Can you work these out from the model? Positions are in its coordinate system, mm. A direction names the side the tool comes from. Coordinates: 2 decimals unless noted, no trailing zeros. Order: outer loops, then holes, each group sorted by start corner. A loop starts at its lowest first (then second) coordinate and runs counter-clockwise, first axis right, second up. Notation, with made-up numbers: (-15.75, -4.5) -> (-6.75, -4.5) arc R17 cw to (-6.75, 9.5) -> close; hole circle Ø6 at (-9, 17.5). An arc over 180 degrees is marked (long way). Answer in a Markdown table with one row per item.
```python
from build123d import *

# Parameters (mm, degrees)
BOSS_EXTRUDE1_DEPTH = 23.622
BOSS_EXTRUDE2_DEPTH = 10.668
SKETCH4_R           = 1.499997
BOSS_EXTRUDE3_DEPTH = 8


with BuildPart() as part:
    # Sketch1 → Boss-Extrude1 (new body)
    with BuildSketch(Plane(origin=(0, 0, 0), x_dir=(1, 0, 0), z_dir=(0, 1, 0))):
        with BuildLine():
            Line((11.557, 4.953), (-11.557, 4.953))
            ThreePointArc((-11.557, 4.953), (-11.916210245, 4.804210245), (-12.065, 4.445))
            Line((-12.065, 4.445), (-12.065, -4.445))
            ThreePointArc((-12.065, -4.445), (-11.916210245, -4.804210245), (-11.557, -4.953))
            Line((-11.557, -4.953), (11.557, -4.953))
            ThreePointArc((11.557, -4.953), (11.916210245, -4.804210245), (12.065, -4.445))
            Line((12.065, -4.445), (12.065, 4.445))
            ThreePointArc((12.065, 4.445), (11.916210245, 4.804210245), (11.557, 4.953))
        make_face()
    extrude(amount=BOSS_EXTRUDE1_DEPTH)

    # Sketch2 → Boss-Extrude2 (add)
    with BuildSketch(Plane(origin=(0, 23.622, 0), x_dir=(1, 0, 0), z_dir=(0, 1, 0))):
        with BuildLine():
            Line((11.557, 4.953), (-11.557, 4.953))
            ThreePointArc((-11.557, 4.953), (-11.916210245, 4.804210245), (-12.065, 4.445))
            Line((-12.065, 4.445), (-12.065, -4.445))
            ThreePointArc((-12.065, -4.445), (-11.916210245, -4.804210245), (-11.557, -4.953))
            Line((-11.557, -4.953), (11.557, -4.953))
            ThreePointArc((11.557, -4.953), (11.916210245, -4.804210245), (12.065, -4.445))
            Line((12.065, -4.445), (12.065, 4.445))
            ThreePointArc((12.065, 4.445), (11.916210245, 4.804210245), (11.557, 4.953))
        make_face()
        with BuildLine():
            Line((10.287, -3.683), (-10.287, -3.683))
            ThreePointArc((-10.287, -3.683), (-10.646210245, -3.534210245), (-10.795, -3.175))
            Line((-10.795, -3.175), (-10.795, 3.175))
            ThreePointArc((-10.795, 3.175), (-10.646210245, 3.534210245), (-10.287, 3.683))
            Line((-10.287, 3.683), (10.287, 3.683))
            ThreePointArc((10.287, 3.683), (10.646210245, 3.534210245), (10.795, 3.175))
            Line((10.795, 3.175), (10.795, -3.175))
            ThreePointArc((10.795, -3.175), (10.646210245, -3.534210245), (10.287, -3.683))
        make_face(mode=Mode.SUBTRACT)
    extrude(amount=BOSS_EXTRUDE2_DEPTH)

    # Sketch4 → Boss-Extrude3 (add)
    with BuildSketch(Plane(origin=(0, 0, 0), x_dir=(1, 0, 0), z_dir=(0, 1, 0))):
        with BuildLine():
            Line((-8.89, -13.184), (8.89, -13.184))
            ThreePointArc((8.89, -13.184), (11.584076836, -12.068076836), (12.7, -9.374))
            Line((12.7, -9.374), (12.7, 9.374))
            ThreePointArc((12.7, 9.374), (11.584076836, 12.068076836), (8.89, 13.184))
            Line((8.89, 13.184), (-8.89, 13.184))
            ThreePointArc((-8.89, 13.184), (-11.584076836, 12.068076836), (-12.7, 9.374))
            Line((-12.7, 9.374), (-12.7, -9.374))
            ThreePointArc((-12.7, -9.374), (-11.584076836, -12.068076836), (-8.89, -13.184))
        make_face()
        with Locations(Location((0, -9.12, 0), (0, 0, 270))):
            Circle(SKETCH4_R, mode=Mode.SUBTRACT)
        with Locations(Location((0, 9.12, 0), (0, 0, 90))):
            Circle(SKETCH4_R, mode=Mode.SUBTRACT)
    extrude(amount=BOSS_EXTRUDE3_DEPTH)


solid = part.part
```
(1) Will these pins go through, and if not, where does the flat tip stop? pin 1 Ø5 at (y, z) = (29.5, 0) entering from +X (3 decimals); pin 2 Ø2.5 at (x, z) = (0, 9.12) entering from -Y; pin 3 Ø2 at (x, z) = (-0.5, 0.5) entering from +Y; pin 4 Ø3 at (x, y) = (-1.5, 29.5) entering from +Z.
Response values:
| item | result |
|---|---|
| pin 1 | x = 12.065 |
| pin 2 | through |
| pin 3 | y = 23.62 |
| pin 4 | z = 4.95 |
(2) Suppose I cut it at A-A (x = 0). Please give me the cut outline in (y, z), and give its area (3 significant figures).
Response values:
| item | result |
|---|---|
| outline | (0, -13.18) -> (8, -13.18) -> (8, -10.62) -> (0, -10.62) -> close; (0, -7.62) -> (8, -7.62) -> (8, -4.95) -> (34.29, -4.95) -> (34.29, -3.68) -> (23.62, -3.68) -> (23.62, 3.68) -> (34.29, 3.68) -> (34.29, 4.95) -> (8, 4.95) -> (8, 7.62) -> (0, 7.62) -> close; (0, 10.62) -> (8, 10.62) -> (8, 13.18) -> (0, 13.18) -> close |
| area | 345 mm2 |
(3) We'd pull the mould along Z, two halves only. Please class faces 1 (the flat face through (0, 21, 4.953)), 2 (the flat face through (10.795, 29, 0)), 3 (the flat face through (-12.7, 4, 0)): +Z half, -Z half, draft (parallel to the pull), parting line (faces both ways), or undercut.
Response values:
| item | result |
|---|---|
| face 1 | +Z half |
| face 2 | undercut |
| face 3 | draft |
(4) On a 3-axis mill with a long thin cutter (end or side, diameter ignored), from which of +Z, -Z, +X, -X, +Y, -Y can I reach the whole of each face in a straight line? I mean faces 4 (the flat face through (0, 21, -4.953)), 5 (the flat face through (12.065, 21, 0)), 6 (the flat face through (0, 23.622, 0)). Say none if no direction works.
Response values:
| item | result |
|---|---|
| face 4 | -Z, +X, -X, +Y |
| face 5 | +Z, -Z, +X, +Y |
| face 6 | +Y |
(5) Suppose I cut it at D-D (x = 7). Please give me the cut outline in (y, z), and give its area (3 significant figures).
Response values:
| item | result |
|---|---|
| outline | (0, -13.18) -> (8, -13.18) -> (8, -4.95) -> (34.29, -4.95) -> (34.29, -3.68) -> (23.62, -3.68) -> (23.62, 3.68) -> (34.29, 3.68) -> (34.29, 4.95) -> (8, 4.95) -> (8, 13.18) -> (0, 13.18) -> close |
| area | 393 mm2 |
(6) Suppose I cut it at B-B (y = 3.5). Please give me the cut outline in (x, z), and give its area (3 significant figures).
Response values:
| item | result |
|---|---|
| outline | (-12.7, -9.37) arc R3.81 ccw to (-8.89, -13.18) -> (8.89, -13.18) arc R3.81 ccw to (12.7, -9.37) -> (12.7, 9.37) arc R3.81 ccw to (8.89, 13.18) -> (-8.89, 13.18) arc R3.81 ccw to (-12.7, 9.37) -> close; hole circle Ø3 at (0, -9.12); hole circle Ø3 at (0, 9.12) |
| area | 643 mm2 |
(7) I need wall thicknesses on line 1 (X direction, y = 3.25, z = -9.12); line 2 (Z direction, x = 9.5, y = 24); line 3 (Z direction, x = 6.5, y = 13). Which ranges of each line are inside material? Lowest first, please. Write a range as [from, to].
Response values:
| item | result |
|---|---|
| line 1 | [-12.7, -1.5], [1.5, 12.7] |
| line 2 | [-4.95, -3.68], [3.68, 4.95] |
| line 3 | [-4.95, 4.95] |
(8) Suppose I cut it at C-C (y = 19). Please give me the cut outline in (x, z) (3 decimals), and give its area (3 significant figures).
Response values:
| item | result |
|---|---|
| outline | (-12.065, -4.445) arc R0.508 ccw to (-11.557, -4.953) -> (11.557, -4.953) arc R0.508 ccw to (12.065, -4.445) -> (12.065, 4.445) arc R0.508 ccw to (11.557, 4.953) -> (-11.557, 4.953) arc R0.508 ccw to (-12.065, 4.445) -> close |
| area | 239 mm2 |
